```python
from build123d import *

# Parameters (mm, degrees)
SKETCH_1_R                     = 24.5
EXTRUDE_1_DEPTH                = 47
CUT_EXTRUDE_2_DEPTH            = 9.5
SKETCH_4_R                     = 10
CUT_EXTRUDE_4_DEPTH            = 7.5
CUT_EXTRUDE_START              = 3.5
SKETCH_5_OUTSIDE_W             = 67.746
SKETCH_5_OUTSIDE_H             = 67.746
SKETCH_5_OUTSIDE_R             = 17
CUT_EXTRUDE_5_DEPTH            = 7
SKETCH_6_R                     = 9
CUT_EXTRUDE_6_DEPTH            = 40.5
CUT_EXTRUDE_10_DEPTH           = 29.5
CUT_EXTRUDE_11_DEPTH           = 21.5
HOLE_WIZARD_2_561_D            = 1.778
HOLE_WIZARD_2_561_DEPTH        = 10.2733
HOLE_WIZARD_2_561_CSINK_D      = 2.54
HOLE_WIZARD_2_561_CSINK_ANGLE  = 110
HOLE_WIZARD_2_561_TIP          = 0.53416509
HOLE_WIZARD_1_0_1_1_AT_2_COUNT = 2
HOLE_WIZARD_1_0_1_1_AT_2_PITCH = 14
CHAMFER_1_SIZE                 = 0.5


with BuildPart() as part:
    # Эскиз1 → Бобышка-Вытянуть1 (new body)
    with BuildSketch(Plane(origin=(0, 0, 0), x_dir=(1, 0, 0), z_dir=(0, 1, 0))):
        Circle(SKETCH_1_R)
    extrude(amount=EXTRUDE_1_DEPTH)

    # Эскиз2 → Вырез-Вытянуть2 (cut)
    with BuildSketch(Plane(origin=(0, 47, 0), x_dir=(1, 0, 0), z_dir=(0, 1, 0))):
        with BuildLine():
            ThreePointArc((21.071307506, 12.5), (0, 24.5), (-21.071307506, 12.5))
            Line((-21.071307506, 12.5), (21.071307506, 12.5))
        make_face()
        with BuildLine():
            Line((21.071307506, -12.5), (-21.071307506, -12.5))
            ThreePointArc((-21.071307506, -12.5), (0, -24.5), (21.071307506, -12.5))
        make_face()
    extrude(amount=-CUT_EXTRUDE_2_DEPTH, mode=Mode.SUBTRACT)

    # Эскиз4 → Вырез-Вытянуть4 (cut)
    with BuildSketch(Plane(origin=(0, 47, 0), x_dir=(1, 0, 0), z_dir=(0, 1, 0))):
        Circle(SKETCH_4_R)
    extrude(amount=-CUT_EXTRUDE_4_DEPTH, mode=Mode.SUBTRACT)

    # Эскиз5 outside → Вырез-Вытянуть5 (cut, through all)
    with BuildSketch(Plane(origin=(0, 37.5, 0), x_dir=(1, 0, 0), z_dir=(0, 1, 0)).offset(CUT_EXTRUDE_START)):
        Rectangle(SKETCH_5_OUTSIDE_W, SKETCH_5_OUTSIDE_H)
        Circle(SKETCH_5_OUTSIDE_R, mode=Mode.SUBTRACT)
    extrude(amount=CUT_EXTRUDE_5_DEPTH, mode=Mode.SUBTRACT)

    # Эскиз6 → Вырез-Вытянуть6 (cut, through all)
    with BuildSketch(Plane(origin=(0, 39.5, 0), x_dir=(1, 0, 0), z_dir=(0, 1, 0))):
        Circle(SKETCH_6_R)
    extrude(amount=-CUT_EXTRUDE_6_DEPTH, mode=Mode.SUBTRACT)

    # Эскиз7 → Вырез-Повернуть1 (revolve, cut)
    with BuildSketch(Plane.XY):
        Polygon((0, 32), (12, 32), (12, 7), (20, 7), (20, 0), (0, 0), align=None)
    revolve(axis=Axis((0, 0, 0), (0, 1, 0)), mode=Mode.SUBTRACT)

    # Эскиз13 → Вырез-Вытянуть10 (cut)
    with BuildSketch(Plane.XZ):
        with BuildLine():
            Line((2.828427125, 9.899494937), (7.071067812, 5.656854249))
            ThreePointArc((7.071067812, 5.656854249), (9.414213562, 0), (7.071067812, -5.656854249))
            Line((7.071067812, -5.656854249), (-2.828427125, -15.556349186))
            ThreePointArc((-2.828427125, -15.556349186), (-8.485281374, -17.899494937), (-14.142135624, -15.556349186))
            Line((-14.142135624, -15.556349186), (-18.384776311, -11.313708499))
            ThreePointArc((-18.384776311, -11.313708499), (-20.727922061, -5.656854249), (-18.384776311, 0))
            Line((-18.384776311, 0), (-8.485281374, 9.899494937))
            ThreePointArc((-8.485281374, 9.899494937), (-2.828427125, 12.242640687), (2.828427125, 9.899494937))
        make_face()
    extrude(amount=-CUT_EXTRUDE_10_DEPTH, mode=Mode.SUBTRACT)

    # Эскиз14 → Вырез-Вытянуть11 (cut)
    with BuildSketch(Plane.XZ):
        with BuildLine():
            Line((9.748922014, 22.476844075), (6.26536991, 18.993291971))
            ThreePointArc((6.26536991, 18.993291971), (14.142135624, 14.142135624), (18.993291971, 6.26536991))
            Line((18.993291971, 6.26536991), (22.476844075, 9.748922014))
            ThreePointArc((22.476844075, 9.748922014), (17.324116139, 17.324116139), (9.748922014, 22.476844075))
        make_face()
        with BuildLine():
            Line((6.26536991, 18.993291971), (-6.363961031, 6.363961031))
            Line((-6.363961031, 6.363961031), (6.363961031, -6.363961031))
            Line((6.363961031, -6.363961031), (18.993291971, 6.26536991))
            ThreePointArc((18.993291971, 6.26536991), (14.142135624, 14.142135624), (6.26536991, 18.993291971))
        make_face()
    extrude(amount=-CUT_EXTRUDE_11_DEPTH, mode=Mode.SUBTRACT)

    # Отверстие обработанное метчиком #2-561
    with Locations(Plane.XZ.offset(-7)):
        with Locations((0, -16.970562748), (16.970562748, 0), (-16.263455967, 5.656854249)):
            CounterSinkHole(HOLE_WIZARD_2_561_D / 2, HOLE_WIZARD_2_561_CSINK_D / 2, depth=HOLE_WIZARD_2_561_DEPTH, counter_sink_angle=HOLE_WIZARD_2_561_CSINK_ANGLE)
            with Locations((0, 0, -(HOLE_WIZARD_2_561_DEPTH + HOLE_WIZARD_2_561_TIP / 2))):  # 118° drill point
                Cone(0, HOLE_WIZARD_2_561_D / 2, HOLE_WIZARD_2_561_TIP, mode=Mode.SUBTRACT)

    # Эскиз23 → Диаметр отверстия Ø1.0 (1)1 (revolve, cut)
    with BuildSketch(Plane(origin=(-7, 41, 12.5), x_dir=(0, -1, 0), z_dir=(1, 0, 0))):
        Polygon((0, 0), (0, 25), (0.525, 25), (0.5, 24.975), (0.5, 0.025), (0.525, 0), align=None)
    hole_wizard_1_0_1_1 = revolve(axis=Axis((-7, 41, 18.85), (0, 0, -1)), mode=Mode.SUBTRACT)

    # Диаметр отверстия Ø1.0 (1)1 at 2: Диаметр отверстия Ø1.0 (1)1 ×2
    with Locations(*[(i * HOLE_WIZARD_1_0_1_1_AT_2_PITCH, 0, 0) for i in range(1, HOLE_WIZARD_1_0_1_1_AT_2_COUNT)]):
        add(hole_wizard_1_0_1_1, mode=Mode.SUBTRACT)

    # Эскиз24 → Вырез-Повернуть2 (revolve, cut)
    with BuildSketch(Plane(origin=(0, 0, 0), x_dir=(0, 0, -1), z_dir=(1, 0, 0))):
        Polygon((24.5, 37.000075506), (24.000075506, 37.5), (24.5, 37.999924494), align=None)
    revolve(axis=Axis((0, 0, 0), (0, 1, 0)), mode=Mode.SUBTRACT)

    # Фаска1
    chamfer_1_edges = [part.edges().sort_by_distance(p)[0] for p in [
        (-20.482902496, 0, -13.442496246),
        (-17, 47, 0),
        (17, 47, 0),
        (-24.5, 41, 0),
        (24.5, 41, 0),
    ]]
    chamfer(chamfer_1_edges, length=CHAMFER_1_SIZE)


solid = part.part
```
Geometry check sheet. Reference: the model listing, model coordinates, mm. A direction names the side the tool comes from. Give positions to 0.01 mm unless a question says otherwise; leave off trailing zeros. Loops run counter-clockwise (first coordinate to the right, second up) from the corner with the lowest first, then second, coordinate; pieces in that order, holes last. Notation, with made-up numbers: (40.25, 56.5) - (46.25, 56.5) arc R25 cw to (46.25, 83.5) - close; hole circle Ø3 at (33, -18). An arc over 180 degrees is marked (long way). Use CSV: the item, a comma, the result in double quotes. Start each with the question number.
Q1. Access from +Z, -Z, +X, -X, +Y, -Y to the whole of each face (thin tool, end or side, straight path). Record for faces 1 (the face through (0, 41, -12.5)), 2 (the face through (17, 44, 0)), 3 (the face through (0, 41, 12.5)), 4 (the face through (-12, 29.5, -9)).
Q2. Section check A-A, the plane y = 27.5. Record the cut outline in (x, z).
Q3. Section check C-C, the plane y = 33. Record the cut outline in (x, z), and give its area (3 significant figures).
Q4. Release check for a two-part mould opening along X. For faces 5 (the face through (24.5, 39.2, 0.2)), 6 (the face through (-17, 44, 0)), 7 (the face through (-16.18, 17.715, 5.787)) record: +X half, -X half, draft (parallel to the pull), parting line (faces both ways), or undercut.
Q5. Go/stop test with flat-tipped pins: pin 1 Ø12 at (x, z) = (0, 0) entering from -Y; pin 2 Ø10 at (x, y) = (16.5, 33.5) entering from -Z; pin 3 Ø23.5 at (x, z) = (0, 0) entering from -Y; pin 4 Ø1 at (y, z) = (25, 7) entering from -X. Record where each tip stops, or that it passes through.
Q6. Scan lines: probe 1 along X at (y, z) = (9, 5.5); probe 2 along Y at (x, z) = (7, 9); probe 3 along Z at (x, y) = (0, 37). Record each from-to range of solid material in increasing order. Write a range as from..to.
Findings below:
1,face 1,"-Z, +X, -X, +Y"
1,face 2,"+X, +Y"
1,face 3,"+Z, +X, -X, +Y"
1,face 4,"-Y"
2,outline,"circle Ø49 at (0, 0); hole (-18.38, -11.31) - (-14.14, -15.56) arc R8 ccw to (-2.83, -15.56) - (0.75, -11.98) arc R12 ccw to (-0.78, 11.97) arc R8 ccw to (-8.49, 9.9) - (-18.38, 0) arc R8 ccw to start"
3,outline,"circle Ø49 at (0, 0); hole circle Ø18 at (0, 0)"
3,area,"1,630 mm^2"
4,face 5,"+X half"
4,face 6,"-X half"
4,face 7,"undercut"
5,pin 1,"passes through"
5,pin 2,"stops at z = -21.63"
5,pin 3,"stops at y = 32"
5,pin 4,"stops at x = -23.62"
6,probe 1,"x = -23.87..-17.14, -15.39..-12.88, 18.23..23.87"
6,probe 2,"y = 32..40.5, 41.5..47"
6,probe 3,"z = -24.5..-9, 9..24.5"
